Design review of the part built by this model. Coordinates are the model's own, in mm. A direction names the side the tool comes from. Give positions to 0.01 mm unless a question says otherwise; leave off trailing zeros. Write each loop counter-clockwise with the first axis right and the second up, starting at its lowest first coordinate (ties: lowest second). Pieces come first, ordered by that corner, then holes.
```python
from build123d import *

# Parameters (mm, degrees)
SKETCH3_R          = 0.593950471
CUT_EXTRUDE1_DEPTH = 1.5
SKETCH4_R          = 0.593950471
CUT_EXTRUDE2_DEPTH = 1.5


with BuildPart() as part:
    # Sketch1 → Revolve1 (revolve)
    with BuildSketch(Plane(origin=(0, 0, 0), x_dir=(1, 0, 0), z_dir=(0, 1, 0)), mode=Mode.PRIVATE) as revolve1_sk:
        with BuildLine():
            add(Edge.make_bspline(
                [(-16, -0.5), (-16.59076322, -0.390621653), (-16.887881425, 0.197649901), (-16.95, 0.906049529)],
                knots=[0, 0, 0, 0, 0.787142654, 0.787142654, 0.787142654, 0.787142654], degree=3))
            Line((-16.95, 0.906049529), (-16.95, 1.5))
            Line((-16.95, 1.5), (0, 1.5))
            Line((0, 1.5), (0, 0))
            Line((0, 0), (-16, 0))
            Line((-16, 0), (-16, -0.5))
        make_face()
    revolve(revolve1_sk.sketch.rotate(Axis((0, 0, -1.5), (-1, 0, 0)), 180), axis=Axis((0, 0, -1.5), (-1, 0, 0)))

    # Sketch3 → Cut-Extrude1 (cut)
    with BuildSketch(Plane.ZY.offset(16.95)):
        Polygon((-0.924807923, 1.001242932), (-2.079505776, 0.998752416), (-2.654697853, -0.002490515), (-2.075192077, -1.001242932), (-0.920494224, -0.998752416), (-0.345302147, 0.002490515), align=None)
        with Locations((-1.5, 0)):
            Circle(SKETCH3_R, mode=Mode.SUBTRACT)
    extrude(amount=-CUT_EXTRUDE1_DEPTH, mode=Mode.SUBTRACT)

    # Sketch4 → Cut-Extrude2 (cut)
    with BuildSketch(Plane.ZY.offset(16.95)):
        with Locations((-1.5, 0)):
            Circle(SKETCH4_R)
    extrude(amount=-CUT_EXTRUDE2_DEPTH, mode=Mode.SUBTRACT)


solid = part.part
```
(1) Tool access review of faces 1 (the face through (0, 0, -2)), 2 (the face through (-16.18, 0.49, -0.63)): name each direction out of +Z, -Z, +X, -X, +Y, -Y from which nothing blocks a thin tool from reaching the whole face with its end or side.
Resolved:
face 1: +Z, -Z, +X, +Y, -Y
face 2: -X
(2) Mouldability with a two-part tool opening along Y and no side actions: class faces 3 (the face through (-8, 0, 0)), 4 (the face through (-16, -1, -3)), 5 (the face through (-16.18, -0.49, -2.37)) as pulls with the +Y half, pulls with the -Y half, needs draft (parallel to the pull), parting line crosses it, or undercut.
Resolved:
face 3: parting line crosses it
face 4: needs draft
face 5: undercut
(3) To check wall thickness, follow L1, parallel to X at y = 0.65, z = -1.25; L2, parallel to Y at x = -7.5, z = -0.85; L3, parallel to Y at x = -12, z = -1.8. State the ranges of each line that lie inside material, in increasing order.
Resolved:
L1: x = -15.45 to 0
L2: y = -1.35 to 1.35
L3: y = -1.47 to 1.47
(4) Consider section A-A, the plane x = -10. Give the boundary of the cut face in (y, z).
Resolved:
outline: circle Ø3 at (0, -1.5)
(5) Clearance check with flat-ended pins moving along their axes: P1, Ø1, axis at x = -2.5, z = -0.5, coming from the +Y side; P2, Ø1, axis at y = 0, z = -1.5, coming from the -X side. State where each tip first meets the part, or that it passes through.
Resolved:
P1: stops at y = 1.41
P2: stops at x = -15.45
